from build123d import *

# Parameters (mm, degrees)
BOSS_EXTRUDE1_DEPTH             = 10
SKETCH2_R                       = 2.85
CUT_EXTRUDE1_DEPTH              = 14
SKETCH5_R                       = 5
CUT_EXTRUDE2_DEPTH              = 5.5
SKETCH7_W                       = 150
SKETCH7_H                       = 20
BOSS_EXTRUDE3_DEPTH             = 10
SKETCH8_W                       = 195
SKETCH8_H                       = 5.029902504
BOSS_EXTRUDE4_DEPTH             = 7.5
BOSS_EXTRUDE5_REACH             = 204.461
BOSS_EXTRUDE5_DIRECTION_2_REACH = 204.461
CUT_EXTRUDE3_REACH              = 204.527
SKETCH10_W                      = 195
SKETCH10_H                      = 7
CUT_EXTRUDE4_DEPTH              = 5
SKETCH11_R                      = 3.175
CUT_EXTRUDE5_DEPTH              = 23
SKETCH12_R                      = 7.5
CUT_EXTRUDE6_DEPTH              = 1.470097496
SKETCH14_W                      = 7.794228634
SKETCH14_H                      = 5.029902504
BOSS_EXTRUDE6_DEPTH             = 1.5
CUT_EXTRUDE7_DEPTH              = 4.5
BOSS_EXTRUDE7_DEPTH             = 5.029902504
LPATTERN4_COUNT                 = 5
LPATTERN4_PITCH                 = 25


with BuildPart() as part:
    # Sketch1 → Boss-Extrude1 (new body)
    with BuildSketch(Plane(origin=(0, 0, 0), x_dir=(1, 0, 0), z_dir=(0, 1, 0))):
        Polygon((45, 18.639610307), (63.639610307, 0), (45, -18.639610307), (18.639610307, -45), (-18.639610307, -45), (-45, -18.639610307), (-45, 18.639610307), (-18.639610307, 45), (18.639610307, 45), align=None)
    extrude(amount=-BOSS_EXTRUDE1_DEPTH)

    # Sketch2 → Cut-Extrude1 (cut)
    with BuildSketch(Plane(origin=(0, 0, 0), x_dir=(1, 0, 0), z_dir=(0, 1, 0))):
        with Locations(Location((-32.664074122, -13.529902504, 0), (0, 0, 270))):
            Circle(SKETCH2_R)
        with Locations(Location((-32.664074122, 13.529902504, 0), (0, 0, 270))):
            Circle(SKETCH2_R)
        with Locations(Location((-13.529902504, 32.664074122, 0), (0, 0, 270))):
            Circle(SKETCH2_R)
        with Locations(Location((13.529902504, 32.664074122, 0), (0, 0, 270))):
            Circle(SKETCH2_R)
        with Locations(Location((32.664074122, 13.529902504, 0), (0, 0, 270))):
            Circle(SKETCH2_R)
        with Locations(Location((32.664074122, -13.529902504, 0), (0, 0, 270))):
            Circle(SKETCH2_R)
        with Locations(Location((13.529902504, -32.664074122, 0), (0, 0, 270))):
            Circle(SKETCH2_R)
        with Locations(Location((-13.529902504, -32.664074122, 0), (0, 0, 270))):
            Circle(SKETCH2_R)
    extrude(amount=-CUT_EXTRUDE1_DEPTH, mode=Mode.SUBTRACT)

    # Sketch5 → Cut-Extrude2 (cut)
    with BuildSketch(Plane(origin=(0, 0, 0), x_dir=(1, 0, 0), z_dir=(0, 1, 0))):
        with Locations(Location((-32.664074122, -13.529902504, 0), (0, 0, 270))):
            Circle(SKETCH5_R)
        with Locations(Location((-32.664074122, 13.529902504, 0), (0, 0, 270))):
            Circle(SKETCH5_R)
        with Locations(Location((-13.529902504, 32.664074122, 0), (0, 0, 270))):
            Circle(SKETCH5_R)
        with Locations(Location((13.529902504, 32.664074122, 0), (0, 0, 270))):
            Circle(SKETCH5_R)
        with Locations(Location((32.664074122, 13.529902504, 0), (0, 0, 270))):
            Circle(SKETCH5_R)
        with Locations(Location((32.664074122, -13.529902504, 0), (0, 0, 270))):
            Circle(SKETCH5_R)
        with Locations(Location((13.529902504, -32.664074122, 0), (0, 0, 270))):
            Circle(SKETCH5_R)
        with Locations(Location((-13.529902504, -32.664074122, 0), (0, 0, 270))):
            Circle(SKETCH5_R)
    extrude(amount=-CUT_EXTRUDE2_DEPTH, mode=Mode.SUBTRACT)

    # Sketch7 → Boss-Extrude3 (add)
    with BuildSketch(Plane(origin=(0, 0, 0), x_dir=(1, 0, 0), z_dir=(0, 1, 0))):
        with Locations((120, 0)):
            Rectangle(SKETCH7_W, SKETCH7_H)
    extrude(amount=-BOSS_EXTRUDE3_DEPTH)

    # Sketch8 → Boss-Extrude4 (add)
    with BuildSketch(Plane(origin=(0, 0, 0), x_dir=(1, 0, 0), z_dir=(0, 1, 0))):
        with Locations((97.5, -6.014951252)):
            Rectangle(SKETCH8_W, SKETCH8_H)
        with Locations((97.5, 6.014951252)):
            Rectangle(SKETCH8_W, SKETCH8_H)
    extrude(amount=BOSS_EXTRUDE4_DEPTH)

    # Boss-Extrude5: up to this face of the body (flat: up to its plane)
    boss_extrude5_end = Plane(part.part.faces().sort_by_distance((124.319805153, -5, -10))[0])
    # Sketch13 → Boss-Extrude5 (add, up to the picked face)
    with BuildSketch(Plane(origin=(0, 0, -8.529902504), x_dir=(-1, 0, 0), z_dir=(0, 0, -1)), mode=Mode.PRIVATE) as boss_extrude5_sk1:
        Polygon((-166.339745962, 3.75), (-170.669872981, 11.25), (-179.330127019, 11.25), (-183.660254038, 3.75), (-183.660254038, -3.75), (-166.339745962, -3.75), align=None)
        Polygon((-168.937822174, 3.75), (-171.968911087, 9), (-178.031088913, 9), (-181.062177826, 3.75), (-178.031088913, -1.5), (-171.968911087, -1.5), align=None, mode=Mode.SUBTRACT)
    boss_extrude5_tool1 = split(extrude(boss_extrude5_sk1.sketch, amount=BOSS_EXTRUDE5_REACH, mode=Mode.PRIVATE), bisect_by=boss_extrude5_end, keep=Keep.BOTH, mode=Mode.PRIVATE)
    boss_extrude5 = boss_extrude5_tool1.solids().sort_by(Axis((168.703241, 7.385436, -8.529903), (0, 0, -1)))[0]
    add(boss_extrude5)

    # Boss-Extrude5 direction 2: up to this face of the body (flat: up to its plane)
    boss_extrude5_direction_2_end = Plane(part.part.faces().sort_by_distance((97.5, 3.75, -3.5))[0])
    # Sketch13 → Boss-Extrude5 direction 2 (add, up to the picked face)
    with BuildSketch(Plane(origin=(0, 0, -8.529902504), x_dir=(-1, 0, 0), z_dir=(0, 0, -1)), mode=Mode.PRIVATE) as boss_extrude5_direction_2_sk1:
        Polygon((-166.339745962, 3.75), (-170.669872981, 11.25), (-179.330127019, 11.25), (-183.660254038, 3.75), (-183.660254038, -3.75), (-166.339745962, -3.75), align=None)
        Polygon((-168.937822174, 3.75), (-171.968911087, 9), (-178.031088913, 9), (-181.062177826, 3.75), (-178.031088913, -1.5), (-171.968911087, -1.5), align=None, mode=Mode.SUBTRACT)
    boss_extrude5_direction_2_tool1 = split(extrude(boss_extrude5_direction_2_sk1.sketch, amount=-BOSS_EXTRUDE5_DIRECTION_2_REACH, mode=Mode.PRIVATE), bisect_by=boss_extrude5_direction_2_end, keep=Keep.BOTH, mode=Mode.PRIVATE)
    boss_extrude5_direction_2 = boss_extrude5_direction_2_tool1.solids().sort_by(Axis((168.703241, 7.385436, -8.529903), (0, 0, 1)))[0]
    add(boss_extrude5_direction_2)

    # Cut-Extrude3: up to this face of the body (flat: up to its plane)
    cut_extrude3_end = Plane(part.part.faces().sort_by_distance((83.441968882, 3.75810856, -8.529902504))[0])
    # Sketch9 → Cut-Extrude3 (cut, up to the picked face)
    with BuildSketch(Plane.XY.offset(8.529902504), mode=Mode.PRIVATE) as cut_extrude3_sk1:
        Polygon((0, 0), (12.990381057, 7.5), (0, 7.5), align=None)
    cut_extrude3_tool1 = split(extrude(cut_extrude3_sk1.sketch, amount=-CUT_EXTRUDE3_REACH, mode=Mode.PRIVATE), bisect_by=cut_extrude3_end, keep=Keep.BOTH, mode=Mode.PRIVATE)
    # Sketch9 → Cut-Extrude3 (cut, up to the picked face)
    with BuildSketch(Plane.XY.offset(8.529902504), mode=Mode.PRIVATE) as cut_extrude3_sk2:
        Polygon((182.009618943, 7.5), (195, 0), (195, 7.5), align=None)
    cut_extrude3_tool2 = split(extrude(cut_extrude3_sk2.sketch, amount=-CUT_EXTRUDE3_REACH, mode=Mode.PRIVATE), bisect_by=cut_extrude3_end, keep=Keep.BOTH, mode=Mode.PRIVATE)
    add(cut_extrude3_tool1.solids().sort_by(Axis((4.330127, 5, 8.529903), (0, 0, -1)))[0], mode=Mode.SUBTRACT)
    add(cut_extrude3_tool2.solids().sort_by(Axis((190.669873, 5, 8.529903), (0, 0, -1)))[0], mode=Mode.SUBTRACT)

    # Sketch10 → Cut-Extrude4 (cut)
    with BuildSketch(Plane(origin=(0, 0, 0), x_dir=(1, 0, 0), z_dir=(0, 1, 0))):
        with Locations((97.5, 0)):
            Rectangle(SKETCH10_W, SKETCH10_H)
    extrude(amount=-CUT_EXTRUDE4_DEPTH, mode=Mode.SUBTRACT)

    # Sketch11 → Cut-Extrude5 (cut)
    with BuildSketch(Plane.XY.offset(8.529902504)):
        with Locations((175, 3.75)):
            Circle(SKETCH11_R)
    cut_extrude5 = extrude(amount=-CUT_EXTRUDE5_DEPTH, mode=Mode.SUBTRACT)

    # Sketch12 → Cut-Extrude6 (cut)
    with BuildSketch(Plane.XY.offset(10)):
        with Locations((175, 3.75)):
            Circle(SKETCH12_R)
    cut_extrude6 = extrude(amount=-CUT_EXTRUDE6_DEPTH, mode=Mode.SUBTRACT)

    # Sketch14 → Boss-Extrude6 (add)
    with BuildSketch(Plane(origin=(0, 7.5, 0), x_dir=(1, 0, 0), z_dir=(0, 1, 0))):
        with Locations((175, 6.014951252)):
            Rectangle(SKETCH14_W, SKETCH14_H)
    boss_extrude6 = extrude(amount=BOSS_EXTRUDE6_DEPTH)

    # Sketch15 → Cut-Extrude7 (cut)
    with BuildSketch(Plane(origin=(0, 0, -10), x_dir=(-1, 0, 0), z_dir=(0, 0, -1))):
        Polygon((-168.937822174, 3.75), (-171.968911087, 9), (-178.031088913, 9), (-181.062177826, 3.75), (-178.031088913, -1.5), (-171.968911087, -1.5), align=None)
    cut_extrude7 = extrude(amount=-CUT_EXTRUDE7_DEPTH, mode=Mode.SUBTRACT)

    # Sketch16 → Boss-Extrude7 (add)
    with BuildSketch(Plane.XY.offset(8.529902504)):
        Polygon((168.504809472, 7.5), (170.669872981, 11.25), (179.330127019, 11.25), (181.495190528, 7.5), align=None)
    boss_extrude7 = extrude(amount=-BOSS_EXTRUDE7_DEPTH)

    # LPattern4: Boss-Extrude5, Boss-Extrude5 direction 2, Cut-Extrude5, Cut-Extrude6, Boss-Extrude6, Cut-Extrude7, Boss-Extrude7 ×5
    with Locations(*[(-i * LPATTERN4_PITCH, 0, 0) for i in range(1, LPATTERN4_COUNT)]):
        add(boss_extrude5)
        add(boss_extrude5_direction_2)
        add(cut_extrude5, mode=Mode.SUBTRACT)
        add(cut_extrude6, mode=Mode.SUBTRACT)
        add(boss_extrude6)
        add(cut_extrude7, mode=Mode.SUBTRACT)
        add(boss_extrude7)


solid = part.part
Verification items for the finished model (mm, model axes). A direction names the side the tool comes from. Coordinates: 2 decimals unless noted, no trailing zeros. Order: outer loops, then holes, each group sorted by start corner. A loop starts at its lowest first (then second) coordinate and runs counter-clockwise, first axis right, second up.
1. Release check for a two-part mould opening along Y. For faces 1 (the face through (6.404, 3.698, 6.05)), 2 (the face through (70.432, 6.338, -7.719)), 3 (the face through (-12.028, -2.712, -27.895)) record: +Y half, -Y half, draft (parallel to the pull), parting line (faces both ways), or undercut.
Results found:
face 1: +Y half
face 2: undercut
face 3: draft
2. Set-up check for faces 4 (the face through (150, -1.5, -8)), 5 (the face through (87, 7.5, -6)), 6 (the face through (105.98, 8.39, -7.52)), 7 (the face through (188, 3, -8.53)), 8 (the face through (-35, -5.5, 16)): record each of +Z, -Z, +X, -X, +Y, -Y from which the full face is reachable in a straight line by a thin tool's end or side.
Results found:
face 4: -Z
face 5: +Z, -Z, +Y
face 6: -Z, +Y
face 7: -Z, +X, +Y
face 8: +Y
3. Sectioned sample at C-C, the plane z = -22. Record the cut outline in (x, y).
Results found:
outline: (-41.64, -10) - (41.64, -10) - (41.64, 0) - (-41.64, 0) - close
4. Sectioned sample at A-A, the plane x = 175. Record the cut outline in (y, z) (3 decimals).
Results found:
outline: (-10, -10) - (-1.5, -10) - (-1.5, -5.5) - (0.575, -5.5) - (0.575, -3.5) - (-5, -3.5) - (-5, 3.5) - (0.575, 3.5) - (0.575, 8.53) - (-3.75, 8.53) - (-3.75, 10) - (-10, 10) - close; (6.925, -5.5) - (9, -5.5) - (9, -10) - (11.25, -10) - (11.25, -3.5) - (6.925, -3.5) - close; (6.925, 3.5) - (11.25, 3.5) - (11.25, 8.53) - (6.925, 8.53) - close
5. Go/stop test with flat-tipped pins: pin 1 Ø10 at (x, y) = (75, 3.75) entering from +Z; pin 2 Ø6 at (x, y) = (160, -6.5) entering from -Z; pin 3 Ø2 at (y, z) = (-4.5, -22) entering from +X. Record where each tip stops, or that it passes through.
Results found:
pin 1: stops at z = 8.53
pin 2: stops at z = -10
pin 3: stops at x = 42.64
6. Scan lines: line 1 (Z direction, x = 151, y = 7.75); line 2 (Z direction, x = 141, y = 5.5); line 3 (Z direction, x = 116, y = -5.75). Record each from-to range of solid material in increasing order.
Results found:
line 1: z = -5.5 to -3.5, 3.5 to 8.53
line 2: z = -8.53 to -3.5, 3.5 to 8.53
line 3: z = -10 to 10
7. Sectioned sample at B-B, the plane x = 87.5. Record the cut outline in (y, z), and give its area (3 significant figures).
Results found:
outline: (-10, -10) - (0, -10) - (0, -8.53) - (7.5, -8.53) - (7.5, -3.5) - (-5, -3.5) - (-5, 3.5) - (7.5, 3.5) - (7.5, 8.53) - (0, 8.53) - (0, 10) - (-10, 10) - close
area: 240 mm2
